```python
from build123d import *

# Parameters (mm, degrees)
SKETCH1_R           = 1
BOSS_EXTRUDE1_DEPTH = 2.5


with BuildPart() as part:
    # Sketch1 → Boss-Extrude1 (new body, symmetric)
    with BuildSketch(Plane(origin=(0, 0, 0), x_dir=(1, 0, 0), z_dir=(0, 1, 0))):
        with BuildLine():
            Line((-2.892231872, 13.10273237), (-8.262783668, -4.799106947))
            ThreePointArc((-8.262783668, -4.799106947), (-8.623679423, -5.31405199), (-9.220609953, -5.511759062))
            Line((-9.220609953, -5.511759062), (-9.476579302, -5.511759062))
            Line((-9.476579302, -5.511759062), (-9.476579302, -7.511759062))
            Line((-9.476579302, -7.511759062), (7.523420698, -7.511759062))
            Line((7.523420698, -7.511759062), (7.523420698, -5.511759062))
            Line((7.523420698, -5.511759062), (7.267451349, -5.511759062))
            ThreePointArc((7.267451349, -5.511759062), (6.670520819, -5.31405199), (6.309625064, -4.799106947))
            Line((6.309625064, -4.799106947), (0.939073269, 13.10273237))
            ThreePointArc((0.939073269, 13.10273237), (-0.976579302, 14.528036599), (-2.892231872, 13.10273237))
        make_face()
        with Locations((-0.976579302, -3.301730431)):
            Circle(SKETCH1_R, mode=Mode.SUBTRACT)
        with Locations((-0.976579302, -0.301730431)):
            Circle(SKETCH1_R, mode=Mode.SUBTRACT)
        with Locations((-0.976579302, 2.698269569)):
            Circle(SKETCH1_R, mode=Mode.SUBTRACT)
        with Locations((-0.976579302, 8.698269569)):
            Circle(SKETCH1_R, mode=Mode.SUBTRACT)
        with Locations((-0.976579302, 11.698269569)):
            Circle(SKETCH1_R, mode=Mode.SUBTRACT)
        with Locations((-0.976579302, 5.698269569)):
            Circle(SKETCH1_R, mode=Mode.SUBTRACT)
    extrude(amount=BOSS_EXTRUDE1_DEPTH, both=True)


solid = part.part
```
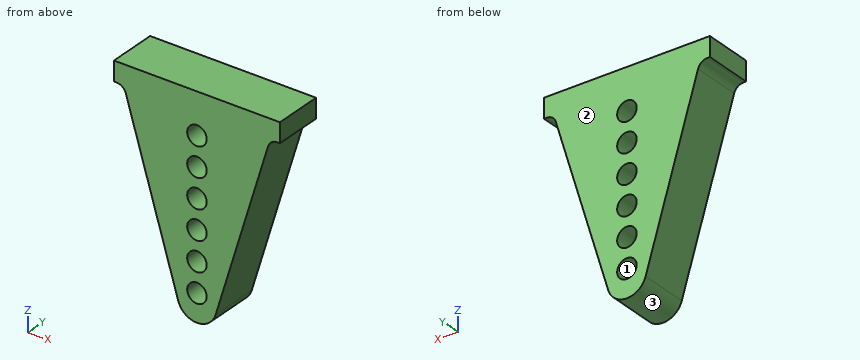
Model file for the job. Use its own axes, mm. Face numbers are marked on the shaded views. Round coordinates to 2 decimals unless told otherwise and drop trailing zeros. Order: outer loops, then holes, each group sorted by start corner. A loop starts at its lowest first (then second) coordinate and runs counter-clockwise, first axis right, second up. Notation, with made-up numbers: M -21,62 L -6,62 A16 cw -6,67 Z; hole C -20,-28 d10. An arc over 180 degrees is marked long. Use CSV: the item, a comma, the result in double quotes.
Item 1: Saw through at B-B (y = 0.8). List the corners of the cut face in (x, z).
Worked answers:
outline,"M -9.48,5.51 L -9.22,5.51 A1 cw -8.26,4.8 L -2.89,-13.1 A2 ccw 0.94,-13.1 L 6.31,4.8 A1 cw 7.27,5.51 L 7.52,5.51 L 7.52,7.51 L -9.48,7.51 Z; hole C -0.98,-11.7 d2; hole C -0.98,-8.7 d2; hole C -0.98,-5.7 d2; hole C -0.98,-2.7 d2; hole C -0.98,0.3 d2; hole C -0.98,3.3 d2"
Item 2: Saw through at C-C (z = -5). List the corners of the cut face in (x, y).
Worked answers:
outline,"M -5.32,-2.5 L -1.69,-2.5 L -1.69,2.5 L -5.32,2.5 Z; M -0.26,-2.5 L 3.37,-2.5 L 3.37,2.5 L -0.26,2.5 Z"
Item 3: Saw through at A-A (z = 3). List the corners of the cut face in (x, y).
Worked answers:
outline,"M -7.72,-2.5 L -1.93,-2.5 L -1.93,2.5 L -7.72,2.5 Z; M -0.02,-2.5 L 5.77,-2.5 L 5.77,2.5 L -0.02,2.5 Z"
Item 4: Pin check, flat tip, straight feed: pin 1 (1.2 mm diameter, centred on x = -0.98, z = -5.7, fed in from +Y). Stop position of the tip, or through.
Worked answers:
pin 1,"through"
Item 5: Pull direction Z, two halves, no side cores. Call the marked faces 1, 2 and 3: released by +Z, released by -Z, zero draft, split by the parting line, or undercut.
Worked answers:
face 1,"undercut"
face 2,"zero draft"
face 3,"released by -Z"
Item 6: Saw through at D-D (x = -3.5). List the corners of the cut face in (y, z).
Worked answers:
outline,"M -2.5,-11.08 L 2.5,-11.08 L 2.5,7.51 L -2.5,7.51 Z"
Item 7: Probe probe 1 along X at (y, z) = (1.9, -2.25); probe 2 along X at (y, z) = (0.95, 0.25); probe 3 along X at (y, z) = (-1.45, -7.5). List the from-to ranges inside material, lowest first.
Worked answers:
probe 1,"-6.15 to -1.87, -0.08 to 4.19"
probe 2,"-6.9 to -1.98, 0.02 to 4.94"
probe 3,"-4.57 to 2.62"
